Autodesk Inventor part; units mm, degrees
ref_plane "YZ Plane" through (0, 0, 0) normal (1, 0, 0) x (0, 1, 0)
ref_plane "XZ Plane" through (0, 0, 0) normal (0, 1, 0) x (-1, 0, 0)
ref_plane "XY Plane" through (0, 0, 0) normal (0, 0, 1) x (1, 0, 0)
sketch "Sketch1" plane through (0, 0, 0) normal (0, 0, 1) x (1, 0, 0)
  circle A0 centre (0, 16) radius 2
  circle A1 centre (-13.8564, -8) radius 2
  circle A2 centre (13.8564, -8) radius 2
  line L0 (0, 28) -> (24.2487, -14)
  line L1 (24.2487, -14) -> (-24.2487, -14)
  line L2 (-24.2487, -14) -> (0, 28)
  circle A3 centre (0, 0) radius 8.1
  line L3 (0, 16) -> (13.8564, -8) construction
  line L4 (13.8564, -8) -> (-13.8564, -8) construction
  line L5 (-13.8564, -8) -> (0, 16) construction
  dimension "d0" = 16.2
  dimension "d1" = 4
  dimension "d2" = 4
  dimension "d3" = 4
  dimension "d4" = 16
  dimension "d5" = 6
extrude "Extrusion1" add sketch "Sketch1" along normal blind 3 contours A0 | A1 | A2 | L0 L1 L2
fillet "Fillet1" radius 6 3 edges at (0, 28, 1.5) (24.2487, -14, 1.5) (-24.2487, -14, 1.5)
sketch "Sketch2" plane through (0, 0, 0) normal (0, 0, -1) x (-1, 0, 0)
  circle A0 centre (0, 0) radius 8.1
  arc A1 (13.8564, -14) -> (19.0526, -5) centre (13.8564, -8) ccw
  line L0 (5.1962, 19) -> (19.0526, -5)
  arc A2 (5.1962, 19) -> (-5.1962, 19) centre (0, 16) ccw
  line L1 (-19.0526, -5) -> (-5.1962, 19)
  arc A3 (-19.0526, -5) -> (-13.8564, -14) centre (-13.8564, -8) ccw
  line L2 (13.8564, -14) -> (-13.8564, -14)
  circle A4 centre (0, 0) radius 11.9
  line L3 (-10.5557, 5.517) -> (-10.0557, 6.383)
  line L4 (-10.0557, 6.383) -> (-6.7514, 4.4753)
  line L5 (-6.7514, 4.4753) -> (-7.2514, 3.6093)
  line L6 (-7.2514, 3.6093) -> (-10.5557, 5.517)
  line L7 (0, 0) -> (-7.0014, 4.0423) construction
  circle A5 centre (0, 0) radius 8.1 construction
  line L8 (-10.0557, 6.383) -> (-11.8744, 7.433)
  line L9 (-10.5557, 5.517) -> (-12.3744, 6.567)
  line L10 (-19.0526, -5) -> (-5.1962, 19)
  line L11 (-13.8744, 3.9689) -> (-11.286, -3.7732)
  line L12 (-10.3744, 10.0311) -> (-2.3753, 11.6605)
  point P0 (-10.3744, 10.0311)
  point P1 (-7.2514, 3.6093)
  point P2 (-12.3744, 6.567)
  point P3 (-13.8744, 3.9689)
  dimension "d9" = 3.8
  dimension "d10" = 1
  dimension "d11" = 3
  dimension "d12" = 3
extrude "Extrusion2" add sketch "Sketch2" along normal blind 8 contours A0 L4 A4 L6 | L4 L8 L1 L12 A4 | A4 L11 L1 L9 L6 picked at (10.5244, -0.9233)
sketch "Sketch3" plane through (6.7514, 4.4753, -8) normal (0.5, -0.8660254, 0) x (0.8660254, 0.5, 0)
  circle A0 centre (2.9577, 4) radius 1.5
  line L0 (0.4577, 5.4434) -> (2.9577, 6.8868)
  line L1 (2.9577, 6.8868) -> (5.4577, 5.4434)
  line L2 (5.4577, 5.4434) -> (5.4577, 2.5566)
  line L3 (5.4577, 2.5566) -> (2.9577, 1.1132)
  line L4 (2.9577, 1.1132) -> (0.4577, 2.5566)
  line L5 (0.4577, 2.5566) -> (0.4577, 5.4434)
  line L6 (5.9154, 8) -> (5.9154, 0)
  line L7 (5.9154, 0) -> (0, 0)
  point P0 (-8.0846, 8)
  point P1 (5.9154, 4)
  point P2 (2.9577, 0)
  dimension "d15" = 3
  dimension "d16" = 5
extrude "Extrusion3" cut sketch "Sketch3" against normal blind 8.75 contours A0 | L0 L1 L2 L3 L4 L5
extrude "Extrusion4" add sketch "Sketch3" against normal blind 3
sketch "Sketch4" plane through (12.3744, 6.567, 0) normal (-0.5, 0.8660254, 0) x (0.8660254, 0.5, 0)
  circle A0 centre (-2.9577, 4) radius 3
  circle A1 centre (-2.9577, 4) radius 1.5
  line L0 (-5.9154, 0) -> (-5.9154, 8)
  line L1 (-5.9154, 8) -> (0, 8)
  line L2 (0, 0) -> (0, 8)
  point P0 (-14, 0)
  point P1 (-5.9154, 4)
  point P2 (-2.9577, 8)
  point P3 (0, 3.4981)
  point P4 (0, 4.5019)
  dimension "d21" = 6
  dimension "d22" = 3
extrude "Extrusion5" cut sketch "Sketch4" against normal through all contours A0 L2 | L2 A0 L0 | L0 A0 | A1
extrude "Extrusion6" add sketch "Sketch4" against normal blind 3 contours L2 A0 L0 | L0 A0 | A1
sketch "Sketch5" plane through (0, 0, 0) normal (0, 0, -1) x (-1, 0, 0)
  line L0 (8.9761, 15.5471) -> (-8.9761, -15.5471)
  line L1 (-7.2514, 3.6093) -> (-12.3744, 6.567)
  line L2 (8.9761, 15.5471) -> (-20.2638, 11.6993)
  line L3 (-20.2638, 11.6993) -> (-8.9761, -15.5471)
  line L4 (0, 0) -> (-20.2638, 11.6993)
  line L5 (-11.8744, 7.433) -> (-6.7514, 4.4753)
extrude "Extrusion7" cut sketch "Sketch5" along normal blind 0.3 contours L0 L4 L2
sketch "Sketch6" plane through (0, 0, 3) normal (0, 0, 1) x (1, 0, 0)
  arc A0 (-19.0526, -5) -> (-13.8564, -14) centre (-13.8564, -8) ccw
  line L0 (-13.8564, -14) -> (13.8564, -14)
  arc A1 (13.8564, -14) -> (19.0526, -5) centre (13.8564, -8) ccw
  line L1 (19.0526, -5) -> (5.1962, 19)
  arc A2 (5.1962, 19) -> (-5.1962, 19) centre (0, 16) ccw
  line L2 (-5.1962, 19) -> (-19.0526, -5)
  circle A3 centre (0, 0) radius 8.1
  line L3 (0, 0) -> (0, 18) construction
  line L4 (0, 0) -> (15.5885, -9) construction
  line L5 (0, 0) -> (-15.5885, -9) construction
  dimension "d32" = 2
  dimension "d33" = 2
  dimension "d34" = 2
hole "Hole1" at (0, 18, 3) at (15.5885, -9, 3) at (-15.5885, -9, 3) direction (0, 0, -1) diameter 3.6 end through all countersink diameter 6.3 countersink angle 90
sketch "Sketch7" plane through (11.3129, 2.49, -4) normal (0.5, -0.8660254, 0) x (0, 0, 1)
  arc A0 (0.5019, -2.9577) -> (-0.5019, -2.9577) centre (0, 0) ccw
  line L0 (-0.5019, -2.9577) -> (0.5019, -2.9577)
  point P0 (4, 11.0423)
hole "Hole2" at (11.3129, 2.49, -4) direction (-0.5, 0.8660254, 0) diameter 2.9 depth 7 tip angle 118
chamfer "Chamfer3" distance 1.5 angle 45 3 edges at (11.1244, 8.7321, -0.3) (11.1244, 8.7321, -8) (13.1244, 5.2679, -8)
equation "\"d33\" = d32"
equation "\"d34\" = d32"
properties part number "Motor Mount Insert"
Build history of the part. All positions in model axes, mm. A direction names the side the tool comes from. Coordinates: 2 decimals unless noted, no trailing zeros. Order: outer loops, then holes, each group sorted by start corner. A loop starts at its lowest first (then second) coordinate and runs counter-clockwise, first axis right, second up. Notation, with made-up numbers: M 84,85 L 95,85 A25 ccw 95,103 Z; hole C -15,70.5 d6. An arc over 180 degrees is marked long. One line per question, with ' | ' between items. Start each with the question number.
1. Flat gauge pins, fed straight in: P1, Ø2, axis at x = -2, z = -2.5, coming from the +Y side; P2, Ø2, axis at x = -12, z = -3.5, coming from the -Y side; P3, Ø3, axis at x = 10.5, z = -6, coming from the -Y side. Where does each tip first touch, or does it go through?
2. Wall check: line 1 along Z through (x, y) = (7, 8.5); line 2 along X through (y, z) = (-9, 0.95); line 3 along X through (y, z) = (6, -4.5). Give the ranges that are in metal, low to high. Write a range as [from, to].
3. Cut at D-D (z = -3). Count the separate pieces of the cut face and the enclosed holes in it, plus the area to 3 significant figures.
4. Cut at B-B (x = 4.5). Write the cut outline in (y, z).
5. Cut at C-C (y = 18). Write the cut outline in (x, z), plus the area to 3 significant figures.
6. Mould opens along Z. For faces 6 (the face through (-12.221, 6.832, 1.479)), 7 (the face through (-1.9, 8.1, -8)), 8 (the face through (4.46, 9.36, -4.02)) say: +Z half, -Z half, draft (parallel to the pull), parting line (faces both ways), or undercut.
7. Tool access for faces 1 (the face through (5.542, 11.015, -6.663)), 2 (the face through (17.346, -8.61, 0.813)), 3 (the face through (10.41, 8.49, -1.06)), 4 (the face through (8.14, 9.895, -1.664)), 5 (the face through (0, 22, 2)): list every direction of +Z, -Z, +X, -X, +Y, -Y with a clear straight run to the whole face (end or side of a thin tool).
8. Cut at A-A (x = 0). Write the cut outline in (y, z).
The answers:
1) P1: stops at y = 11.86 | P2: stops at y = -4.54 | P3: stops at y = -7.79
2) line 1: z = [-8, -6.47], [-1.53, -0.3], [0, 3] | line 2: x = [-19.77, -17.39], [-13.79, 13.79], [17.39, 19.77] | line 3: x = [-10.28, -5.44], [5.44, 7.65], [11.39, 12.7]
3) separate pieces: 3 | enclosed holes: 0 | area: 218 mm2
4) outline: M -14,0 L -11.02,0 L -11.02,-8 L -6.73,-8 L -6.73,3 L -14,3 Z; M 6.73,-8 L 11.23,-8 L 11.23,-6 L 9.29,-5.44 L 9.29,-2.56 L 11.23,-2 L 11.23,-0.3 L 6.73,-0.3 Z; M 6.73,0 L 19.97,0 L 19.97,3 L 6.73,3 Z
5) outline: M -5.77,0 L -1.8,0 L -1.8,1.65 L -3.15,3 L -5.77,3 Z; M 1.8,0 L 5.77,0 L 5.77,3 L 3.15,3 L 1.8,1.65 Z | area: 22.0 mm2
6) face 6: draft | face 7: -Z half | face 8: undercut
7) face 1: -Z, +X, +Y | face 2: +Z, -Z | face 3: +X, +Y | face 4: none | face 5: +Z, -Z, +Y
8) outline: M -14,0 L -11.9,0 L -11.9,-8 L -8.1,-8 L -8.1,3 L -14,3 Z; M 8.1,-8 L 11.9,-8 L 11.9,-0.3 L 8.1,-0.3 Z; M 8.1,0 L 16.2,0 L 16.2,1.65 L 14.85,3 L 8.1,3 Z; M 19.8,0 L 22,0 L 22,3 L 21.15,3 L 19.8,1.65 Z
